Input: part model. Units: mm. Frame: model coordinates. Face numbers are marked on the shaded views. A direction names the side the tool comes from. Give positions to 0.01 mm unless a question says otherwise; leave off trailing zeros. Write each loop counter-clockwise with the first axis right and the second up, starting at its lowest first coordinate (ties: lowest second). Pieces come first, ordered by that corner, then holes. Notation, with made-up numbers: (55.5, 42.5) - (87.5, 42.5) arc R8 ccw to (87.5, 55.5) - close; hole circle Ø6 at (5.5, 52). An arc over 180 degrees is marked (long way). Answer as a JSON object with one key per item and string values. Group by question number.
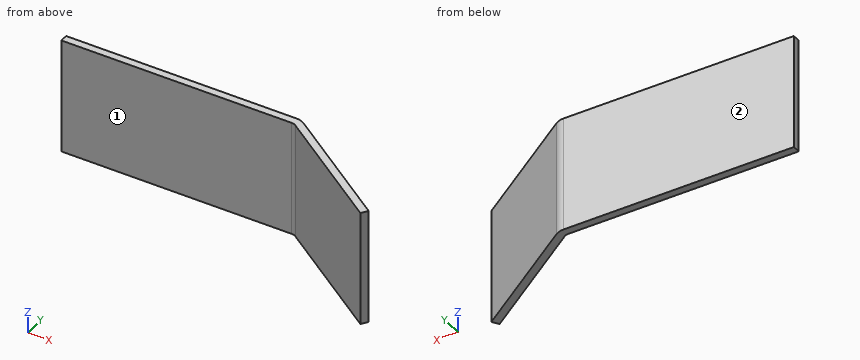
from build123d import *

# Parameters (mm, degrees)
SM_BASE_FLANGE_1_DEPTH = 60
CUT_EXTRUDE_1_DEPTH    = 306.076680355


# Sheet-metal steps are written as plain solids
with BuildPart() as part:
    # Sketch 1 → 基体-法兰1 (new, symmetric)
    with BuildSketch(Plane.XY):
        with BuildLine():
            Line((-245, 0), (-5.044780622, 0))
            ThreePointArc((-5.044780622, 0), (-0.23348783, -0.740528788), (4.13244236, -2.893567291))
            Line((4.13244236, -2.893567291), (185.659240876, -130))
            Line((185.659240876, -130), (181.070629386, -136.553216354))
            Line((181.070629386, -136.553216354), (-0.456169131, -9.446783646))
            ThreePointArc((-0.456169131, -9.446783646), (-2.639134226, -8.370264394), (-5.044780622, -8))
            Line((-5.044780622, -8), (-245, -8))
            Line((-245, -8), (-245, 0))
        make_face()
    extrude(amount=SM_BASE_FLANGE_1_DEPTH, both=True)

    # 草图6 → 切除-拉伸1 (cut, through all)
    with BuildSketch(Plane.XY.offset(60)):
        Polygon((124.248876587, -87), (119.660265096, -93.553216354), (181.070629386, -136.553216354), (185.659240876, -130), align=None)
    extrude(amount=-CUT_EXTRUDE_1_DEPTH, mode=Mode.SUBTRACT)


solid = part.part
1) Cut plane C-C on y = -62.5. Return the cut outline in (x, z), and give its area (3 significant figures).
2) Cut plane A-A on z = 52. Return the cut outline in (x, y), and give its area (3 significant figures).
3) Pin query (flat end, axial travel): P1, Ø2, axis at y = -76, z = 1.5, coming from the +X side; P2, Ø2, axis at x = -63, z = 46.5, coming from the -Y side; P3, Ø2, axis at x = 47, z = 12.5, coming from the +Y side. Return the tip coordinate at first contact, or that it passes through.
4) Cut plane B-B on x = -70. Return the cut outline in (y, z).
5) Reachability of the marked faces 1 and 2 from +Z, -Z, +X, -X, +Y, -Y: full face, straight path, thin tool, end or side. Return the list, or none.
6) Line query: line 1 along Y through (x, z) = (-67, 14.5); line 2 along X through (y, z) = (-78, 20); line 3 along X through (y, z) = (-17.5, -40). Output: solid intervals per line, ascending. Write a range as from..to.
Filled in:
{
 "1": {"outline": "(75.31, -60) - (89.26, -60) - (89.26, 60) - (75.31, 60) - close", "area": "1,670 mm²"},
 "2": {"outline": "(-245, -8) - (-5.04, -8) arc R8 cw to (-0.46, -9.45) - (119.66, -93.55) - (124.25, -87) - (4.13, -2.89) arc R16 ccw to (-5.04, 0) - (-245, 0) - close", "area": "3,150 mm²"},
 "3": {"P1": "stops at x = 109.97", "P2": "stops at y = -8", "P3": "stops at y = -32.21"},
 "4": {"outline": "(-8, -60) - (0, -60) - (0, 60) - (-8, 60) - close"},
 "5": {"face 1": "+Z, -Z, -X, -Y", "face 2": "+Z, -Z, +X, -X, +Y"},
 "6": {"line 1": "y = -8..0", "line 2": "x = 97.45..111.4", "line 3": "x = 11.05..24.99"}
}
